The model under review builds one solid part; all positions refer to its coordinate system, in mm. Face numbers are marked on the shaded views. A direction names the side the tool comes from. Give positions to 0.01 mm unless a question says otherwise; leave off trailing zeros. Loops run counter-clockwise (first coordinate to the right, second up) from the corner with the lowest first, then second, coordinate; pieces in that order, holes last. Notation, with made-up numbers: M -34,87 L 8,87 A14 cw 8,99 Z; hole C 9,41 d5. An arc over 180 degrees is marked long. Put each result on its own line as item: value. Start each with the question number.
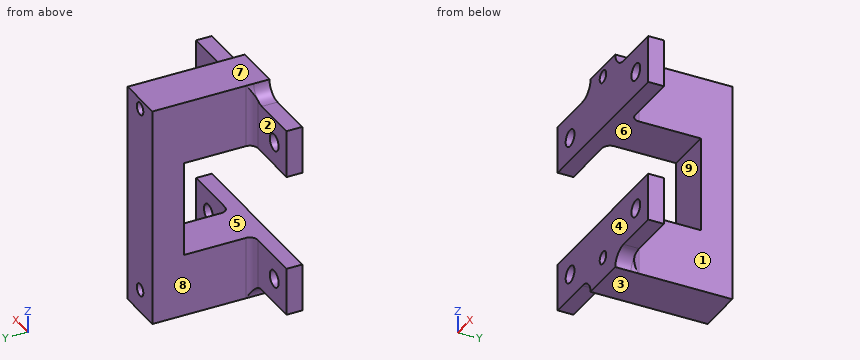
```python
from build123d import *

# Parameters (mm, degrees)
BOSS_EXTRUDE1_DEPTH         = 4.7625
SKETCH4_W                   = 12.7
SKETCH4_H                   = 9.652
BOSS_EXTRUDE2_DEPTH         = 3.175
M3_CLEARANCE_HOLE1_D        = 3.4
MIRROR2_COPY_1_SKETCH_W     = 12.7
MIRROR2_COPY_1_SKETCH_H     = 9.652
MIRROR2_COPY_1_DEPTH        = 3.175
MIRROR2_COPY_2_D            = 3.4
FILLET1_R                   = 3.175
FILLET2_R                   = 1.5875
TAP_DRILL_FOR_M3X0_5_TAP1_D = 2.5


with BuildPart() as part:
    # Sketch2 → Boss-Extrude1 (new, symmetric)
    with BuildSketch(Plane(origin=(0, 0, 0), x_dir=(0, 0, -1), z_dir=(1, 0, 0))):
        Polygon((22.352, 23.622), (-22.352, 23.622), (-22.352, 0), (-9.652, 0), (-9.652, 17.272), (9.652, 17.272), (9.652, 0), (22.352, 0), align=None)
    extrude(amount=BOSS_EXTRUDE1_DEPTH, both=True)

    # Sketch4 → Boss-Extrude2 (add)
    with BuildSketch(Plane.XZ):
        with Locations((11.1125, 14.478)):
            Rectangle(SKETCH4_W, SKETCH4_H)
    boss_extrude2 = extrude(amount=-BOSS_EXTRUDE2_DEPTH)

    # M3 Clearance Hole1 (through all)
    with Locations(Plane(origin=(0, 3.175, 0), x_dir=(1, 0, 0), z_dir=(0, 1, 0))):
        with Locations((12.7, -14.351)):
            m3_clearance_hole1 = Hole(M3_CLEARANCE_HOLE1_D / 2)

    # Mirror1: Boss-Extrude2, M3 Clearance Hole1 across plane
    add(boss_extrude2.mirror(Plane.XY))
    add(m3_clearance_hole1.mirror(Plane.XY), mode=Mode.SUBTRACT)

    # Mirror2: Boss-Extrude2, M3 Clearance Hole1 across plane
    add(boss_extrude2.mirror(Plane(origin=(0, 0, 0), x_dir=(0, 0, 1), z_dir=(1, 0, 0))))
    add(m3_clearance_hole1.mirror(Plane(origin=(0, 0, 0), x_dir=(0, 0, 1), z_dir=(1, 0, 0))), mode=Mode.SUBTRACT)

    # Mirror2 copy 1 sketch → Mirror2 copy 1 (add)
    with BuildSketch(Plane(origin=(0, 0, 0), x_dir=(-1, 0, 0), z_dir=(0, -1, 0))):
        with Locations((11.1125, 14.478)):
            Rectangle(MIRROR2_COPY_1_SKETCH_W, MIRROR2_COPY_1_SKETCH_H)
    extrude(amount=-MIRROR2_COPY_1_DEPTH)

    # Mirror2 copy 2 (through all)
    with Locations(Plane(origin=(0, 3.175, 0), x_dir=(-1, 0, 0), z_dir=(0, 1, 0))):
        with Locations((12.7, -14.351)):
            Hole(MIRROR2_COPY_2_D / 2)

    # Fillet1
    # the kernel refuses this fillet: 3.175 mm, written as the material it adds along each edge
    with BuildSketch(Plane(origin=(-4.7625, 0, -19.304), x_dir=(0, 0, -1), z_dir=(0, 1, 0)), Plane(origin=(4.7625, 0, 19.304), x_dir=(0, 0, 1), z_dir=(0, 1, 0))) as fillet1_piece_1:
        with BuildLine():
            CenterArc((3.175, 3.172458983), FILLET1_R, 180, 87.707557224)
            Line((0, 3.172458983), (-0.0635, 3.172458983))
            Line((-0.0635, 3.172458983), (-0.0635, 0))
            Line((-0.0635, 0), (0, -0.0635))
            ThreePointArc((0, -0.0635), (1.524, -0.0635), (3.04546, -0.06344918))
            Line((3.04546, -0.06344918), (3.048, 0))
        make_face()
    extrude(amount=3.175)
    with BuildSketch(Plane(origin=(4.7625, 0, -19.304), x_dir=(0, 0, -1), z_dir=(0, 1, 0)), Plane(origin=(-4.7625, 0, 19.304), x_dir=(0, 0, 1), z_dir=(0, 1, 0))) as fillet1_piece_2:
        with BuildLine():
            CenterArc((3.175, -3.172458983), FILLET1_R, 92.292442776, 87.707557224)
            Line((0, -3.172458983), (-0.0635, -3.172458983))
            Line((-0.0635, -3.172458983), (-0.0635, 0))
            Line((-0.0635, 0), (0, 0.0635))
            ThreePointArc((0, 0.0635), (1.524, 0.0635), (3.04546, 0.06344918))
            Line((3.04546, 0.06344918), (3.048, 0))
        make_face()
    extrude(amount=3.175)

    # Fillet2
    # the kernel refuses this fillet: 1.5875 mm, written as the material it adds along each edge
    with BuildSketch(Plane(origin=(4.7625, 3.175, 22.352), x_dir=(1, 0, 0), z_dir=(0, 0, -1))) as fillet2_piece_1_section:
        with BuildLine():
            CenterArc((FILLET2_R, -FILLET2_R), FILLET2_R, 90, 90)
            Line((0, -FILLET2_R), (0, 0))
            Line((0, 0), (FILLET2_R, 0))
        make_face()
    fillet2_piece_1 = extrude(amount=12.7, mode=Mode.PRIVATE)
    fillet2_piece_1 = fillet2_piece_1 - Plane(origin=(7.934958983, 3.539048881, 22.479), x_dir=(0, 0, 1), z_dir=(0, -1, 0)) * Cylinder(3.175, 32, mode=Mode.PRIVATE)
    add(fillet2_piece_1)
    with BuildSketch(Plane(origin=(4.7625, 3.175, -22.352), x_dir=(1, 0, 0), z_dir=(0, 0, 1))) as fillet2_piece_2_section:
        with BuildLine():
            CenterArc((FILLET2_R, FILLET2_R), FILLET2_R, 180, 90)
            Line((0, FILLET2_R), (0, 0))
            Line((0, 0), (FILLET2_R, 0))
        make_face()
    fillet2_piece_2 = extrude(amount=12.7, mode=Mode.PRIVATE)
    fillet2_piece_2 = fillet2_piece_2 - Plane(origin=(7.934958983, 3.539054825, -22.479), x_dir=(0, 0, -1), z_dir=(0, -1, 0)) * Cylinder(3.175, 32, mode=Mode.PRIVATE)
    add(fillet2_piece_2)
    with BuildSketch(Plane(origin=(-4.7625, 3.175, 9.652), x_dir=(0, 1, 0), z_dir=(0, 0, 1))) as fillet2_piece_3_section:
        with BuildLine():
            CenterArc((FILLET2_R, FILLET2_R), FILLET2_R, 180, 90)
            Line((0, FILLET2_R), (0, 0))
            Line((0, 0), (FILLET2_R, 0))
        make_face()
    fillet2_piece_3 = extrude(amount=12.7, mode=Mode.PRIVATE)
    fillet2_piece_3 = fillet2_piece_3 - Plane(origin=(-7.934958983, 3.539056273, 22.479), x_dir=(0, 0, 1), z_dir=(0, -1, 0)) * Cylinder(3.175, 32, mode=Mode.PRIVATE)
    add(fillet2_piece_3)
    with BuildSketch(Plane(origin=(-4.7625, 3.175, -9.652), x_dir=(-1, 0, 0), z_dir=(0, 0, -1))) as fillet2_piece_4_section:
        with BuildLine():
            CenterArc((FILLET2_R, FILLET2_R), FILLET2_R, 180, 90)
            Line((0, FILLET2_R), (0, 0))
            Line((0, 0), (FILLET2_R, 0))
        make_face()
    fillet2_piece_4 = extrude(amount=12.7, mode=Mode.PRIVATE)
    fillet2_piece_4 = fillet2_piece_4 - Plane(origin=(-7.934958983, 3.539048881, -22.479), x_dir=(0, 0, -1), z_dir=(0, -1, 0)) * Cylinder(3.175, 32, mode=Mode.PRIVATE)
    add(fillet2_piece_4)

    # Tap Drill for M3x0.5 Tap1 (through all)
    with Locations(Plane(origin=(0, 23.622, 0), x_dir=(1, 0, 0), z_dir=(0, 1, 0))):
        with Locations((0, 17.778984556), (0, -20.321015444)):
            Hole(TAP_DRILL_FOR_M3X0_5_TAP1_D / 2)


solid = part.part
```
Item 1: Consider section D-D, the plane x = 12.7. Write out the cut boundary in (y, z) (3 decimals), plus the area to 3 significant figures.
Item 2: Consider section B-B, the plane y = 6.5. Write out the cut boundary in (x, z).
Item 3: Draft analysis for pull direction Z (two halves, no side actions). For the marked faces 6, 7, 8 and 9, state which applies: +Z half, -Z half, draft (parallel to the pull), parting line (faces both ways), or undercut.
Item 4: Consider section C-C, the plane x = 9. Write out the cut boundary in (y, z) (3 decimals).
Item 5: To check wall thickness, follow L1, parallel to Z at x = 12.7, y = 1.65; L2, parallel to Z at x = 3, y = 11; L3, parallel to Z at x = 0, y = 5.25. State the ranges of each line that lie inside material, in increasing order. Write a range as [from, to].
Item 6: Clearance check with flat-ended pins moving along their axes: pin 1 Ø1.6 at (x, y) = (15, 2) entering from -Z; pin 2 Ø4.5 at (x, z) = (-12.7, -14.351) entering from +Y (3 decimals); pin 3 Ø7.5 at (x, z) = (2, -3) entering from -Y. State where each tip first meets the part, or that it passes through.
Item 7: Consider section A-A, the plane x = 0. Write out the cut boundary in (y, z).
Item 8: Tool access review of the marked faces 1, 2, 3, 4 and 5: name each direction out of +Z, -Z, +X, -X, +Y, -Y from which nothing blocks a thin tool from reaching the whole face with its end or side.
Report:
1. outline: M 0,-19.304 L 3.175,-19.304 L 3.175,-16.051 L 0,-16.051 Z; M 0,-12.651 L 3.175,-12.651 L 3.175,-9.652 L 0,-9.652 Z; M 0,9.652 L 3.175,9.652 L 3.175,12.651 L 0,12.651 Z; M 0,16.051 L 3.175,16.051 L 3.175,19.304 L 0,19.304 Z
1. area: 39.7 mm²
2. outline: M -4.76,-22.35 L 4.76,-22.35 L 4.76,-9.65 L -4.76,-9.65 Z; M -4.76,9.65 L 4.76,9.65 L 4.76,22.35 L -4.76,22.35 Z; hole C 0,-17.78 d2.5; hole C 0,20.32 d2.5
3. face 6: undercut
3. face 7: +Z half
3. face 8: draft
3. face 9: undercut
4. outline: M 0,-19.304 L 3.175,-19.304 L 3.175,-9.652 L 0,-9.652 Z; M 0,9.652 L 3.175,9.652 L 3.175,19.304 L 0,19.304 Z
5. L1: [-19.3, -16.05], [-12.65, -9.65], [9.65, 12.65], [16.05, 19.3]
5. L2: [-22.35, -9.65], [9.65, 22.35]
5. L3: [-22.35, -19.03], [-16.53, -9.65], [9.65, 19.07], [21.57, 22.35]
6. pin 1: z = -19.3
6. pin 2: y = 3.175
6. pin 3: y = 17.27
7. outline: M 0,-22.35 L 23.62,-22.35 L 23.62,-19.03 L 0,-19.03 Z; M 0,-16.53 L 23.62,-16.53 L 23.62,19.07 L 0,19.07 L 0,9.65 L 17.27,9.65 L 17.27,-9.65 L 0,-9.65 Z; M 0,21.57 L 23.62,21.57 L 23.62,22.35 L 0,22.35 Z
8. face 1: +Z, -Z, +X, +Y
8. face 2: +Z, -Z, -X, +Y
8. face 3: -Z, +X, -X, +Y, -Y
8. face 4: +Z, -Z, +X, -X, -Y
8. face 5: +X, -X, -Y
